Model file for the job. Use its own axes, mm. Face numbers are marked on the shaded views. Coordinates: 2 decimals unless noted, no trailing zeros. Order: outer loops, then holes, each group sorted by start corner. A loop starts at its lowest first (then second) coordinate and runs counter-clockwise, first axis right, second up. Notation, with made-up numbers: (-35.5, 33) -> (-2.5, 33) arc R25 ccw to (-2.5, 58) -> close; hole circle Ø9 at (-4.5, 62.25). An arc over 180 degrees is marked (long way). Return JSON: item names as keys, results as strings. Group by question number.
1) Pull direction X, two halves, no side cores. Call the marked faces 1, 2 and 3: +X half, -X half, draft (parallel to the pull), parting line (faces both ways), or undercut.
2) Probe line 1 (Y direction, x = 50.8, z = 2.25); line 2 (X direction, y = 25.5, z = 0.75); line 3 (X direction, y = 27.5, z = 5.25). List the from-to ranges inside material, lowest first.
3) Cut at C-C (z = 5.25). Write the cut outline in (x, y).
4) Cut at B-B (y = 25.4). Write the cut outline in (x, z), and give its area (3 significant figures).
5) Cut at A-A (x = 50.8). Write the cut outline in (y, z).
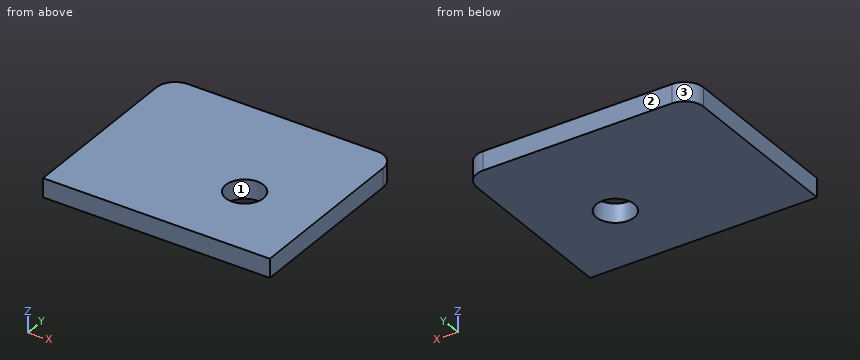
from build123d import *

# Parameters (mm, degrees)
SKETCH1_W           = 76.2
SKETCH1_H           = 63.5
BOSS_EXTRUDE1_DEPTH = 6.35
FILLET1_R           = 6.35
FILLET2_R           = 6.35
SKETCH2_R           = 6.35
CUT_EXTRUDE1_DEPTH  = 7.35


with BuildPart() as part:
    # Sketch1 → Boss-Extrude1 (new body)
    with BuildSketch(Plane.XY):
        with Locations((38.1, 31.75)):
            Rectangle(SKETCH1_W, SKETCH1_H)
    extrude(amount=BOSS_EXTRUDE1_DEPTH)

    # Fillet1
    fillet1_edges = [part.edges().sort_by_distance(p)[0] for p in [
        (0, 63.5, 3.175),
    ]]
    fillet(fillet1_edges, radius=FILLET1_R)

    # Fillet2
    fillet2_edges = [part.edges().sort_by_distance(p)[0] for p in [
        (76.2, 63.5, 3.175),
    ]]
    fillet(fillet2_edges, radius=FILLET2_R)

    # Sketch2 → Cut-Extrude1 (cut, through all)
    with BuildSketch(Plane.XY.offset(6.35)):
        with Locations((50.8, 25.4)):
            Circle(SKETCH2_R)
    extrude(amount=-CUT_EXTRUDE1_DEPTH, mode=Mode.SUBTRACT)


solid = part.part
Answers below:
{
 "1": {"face 1": "undercut", "face 2": "draft", "face 3": "-X half"},
 "2": {"line 1": "y = 0 to 19.05, 31.75 to 63.5", "line 2": "x = 0 to 44.45, 57.15 to 76.2", "line 3": "x = 0 to 44.81, 56.79 to 76.2"},
 "3": {"outline": "(0, 0) -> (76.2, 0) -> (76.2, 57.15) arc R6.35 ccw to (69.85, 63.5) -> (6.35, 63.5) arc R6.35 ccw to (0, 57.15) -> close; hole circle Ø12.7 at (50.8, 25.4)"},
 "4": {"outline": "(0, 0) -> (44.45, 0) -> (44.45, 6.35) -> (0, 6.35) -> close; (57.15, 0) -> (76.2, 0) -> (76.2, 6.35) -> (57.15, 6.35) -> close", "area": "403 mm^2"},
 "5": {"outline": "(0, 0) -> (19.05, 0) -> (19.05, 6.35) -> (0, 6.35) -> close; (31.75, 0) -> (63.5, 0) -> (63.5, 6.35) -> (31.75, 6.35) -> close"}
}
